```python
from build123d import *

# Parameters (mm, degrees)
F0_W      = 68.1
F0_H      = 138.3
F1_DEPTH  = 5.08
F2_R      = 8.93259
F3_T      = -1.15
F4_W      = 24.09836
F4_H      = 13.196725
F5_DEPTH  = 12.5
F6_W      = 48.097777
F6_H      = 7.753484
F7_DEPTH  = 12.5
F8_W      = 10.118616
F8_H      = 41.666549
F9_DEPTH  = 12.5
F10_W     = 6.856616
F10_H     = 19.977162
F11_DEPTH = 12.5
F12_SIZE  = 5


with BuildPart() as f1:
    # F0 (on Front) → F1 (new body, symmetric)
    with BuildSketch(Plane.XZ):
        Rectangle(F0_W, F0_H)
    extrude(amount=F1_DEPTH, both=True)

    # F2
    f2_edges = [f1.edges().sort_by_distance(p)[0] for p in [
        (-34.05, 0, 69.15),
        (34.05, 0, 69.15),
        (34.05, 0, -69.15),
        (-34.05, 0, -69.15),
    ]]
    fillet(f2_edges, radius=F2_R)

    # F3
    f3_openings = [f1.faces().sort_by_distance(p)[0] for p in [
        (0, -5.08, 0),
    ]]
    offset(amount=F3_T, openings=f3_openings)

    # F4 (on face) → F5 (cut, symmetric)
    with BuildSketch(Plane.XZ):
        with Locations((15.348363, 59.815576)):
            Rectangle(F4_W, F4_H)
    extrude(amount=F5_DEPTH, both=True, mode=Mode.SUBTRACT)

    # F6 (on face) → F7 (cut, symmetric)
    with BuildSketch(Plane(origin=(0, 0, -69.15), x_dir=(1, 0, 0), z_dir=(0, 0, -1))):
        with Locations((0.003194, 0.064824)):
            Rectangle(F6_W, F6_H)
    extrude(amount=F7_DEPTH, both=True, mode=Mode.SUBTRACT)

    # F8 (on face) → F9 (cut, symmetric)
    with BuildSketch(Plane(origin=(-34.05, 0, 0), x_dir=(0, -1, 0), z_dir=(-1, 0, 0))):
        with Locations((3.675346, 37.227889)):
            Rectangle(F8_W, F8_H)
    extrude(amount=F9_DEPTH, both=True, mode=Mode.SUBTRACT)

    # F10 (on face) → F11 (cut, symmetric)
    with BuildSketch(Plane.YZ.offset(34.05)):
        with Locations((-1.651692, 39.359077)):
            Rectangle(F10_W, F10_H)
    extrude(amount=F11_DEPTH, both=True, mode=Mode.SUBTRACT)

    # F12
    f12_edges = [f1.edges().sort_by_distance(p)[0] for p in [
        (3.299183, 4.505, 66.413939),
        (27.397543, 4.505, 66.413939),
        (27.397543, 4.505, 53.217214),
        (3.299183, 4.505, 53.217214),
    ]]
    chamfer(f12_edges, length=F12_SIZE)


solid = f1.part
```
Geometry check sheet. Reference: the model listing, model coordinates, mm. A direction names the side the tool comes from. Give positions to 0.01 mm unless a question says otherwise; leave off trailing zeros. Write each loop counter-clockwise with the first axis right and the second up, starting at its lowest first coordinate (ties: lowest second). Pieces come first, ordered by that corner, then holes. Notation, with made-up numbers: (2.25, 11.25) - (48.25, 11.25) arc R17 ccw to (48.25, 42.25) - close; hole circle Ø5 at (43.25, 46). An arc over 180 degrees is marked (long way). Use a Markdown table: item, result.
Q1. Thickness scan on L1, parallel to X at y = 2.25, z = 2; L2, parallel to Z at x = 15, y = -1.75; L3, parallel to Y at x = 10.5, z = 48. Record the ranges inside material, lowest first. Write a range as [from, to].
Computed:
| item | result |
|---|---|
| L1 | x = [-34.05, -32.9], [32.9, 34.05] |
| L2 | z = [68, 69.15] |
| L3 | y = [3.93, 5.08] |
Q2. Section check B-B, the plane x = -19. Enter the section's corners in (y, z), then the cut area to 3 significant figures.
Computed:
| item | result |
|---|---|
| outline | (-5.08, -69.15) - (-3.94, -69.15) - (-3.94, -68) - (-5.08, -68) - close; (-5.08, 68) - (3.93, 68) - (3.93, -68) - (3.81, -68) - (3.81, -69.15) - (5.08, -69.15) - (5.08, 69.15) - (-5.08, 69.15) - close |
| area | 171 mm² |
Q3. Section check D-D, the plane z = -39.5. Enter the section's corners in (x, y), then the cut area to 3 significant figures.
Computed:
| item | result |
|---|---|
| outline | (-34.05, -5.08) - (-32.9, -5.08) - (-32.9, 3.93) - (32.9, 3.93) - (32.9, -5.08) - (34.05, -5.08) - (34.05, 5.08) - (-34.05, 5.08) - close |
| area | 99.0 mm² |
Q4. Go/stop test with flat-tipped pins: P1, Ø0.9, axis at x = -33.5, y = -0.5, coming from the -Z side; P2, Ø0.9, axis at x = -33.5, z = 47.5, coming from the -Y side; P3, Ø1.3, axis at y = 4.5, z = 60.5, coming from the +X side; P4, Ø0.6, axis at x = 33.5, z = 40, coming from the -Y side. Record where each tip stops, or that it passes through.
Computed:
| item | result |
|---|---|
| P1 | stops at z = -64.32 |
| P2 | stops at y = 1.38 |
| P3 | stops at x = 34.05 |
| P4 | stops at y = 1.78 |
Q5. Draft check along X on faces 4 (the face through (0, 3.93, 1)), 5 (the face through (24.93, 4.51, 55.75)), 6 (the face through (-0.1, -4.2, -69.15)), 7 (the face through (-31.503, -0.071, -66.464)). Enter one of: pulls with the +X half, pulls with the -X half, needs draft (parallel to the pull), parting line crosses it, or undercut.
Computed:
| item | result |
|---|---|
| face 4 | undercut |
| face 5 | undercut |
| face 6 | needs draft |
| face 7 | pulls with the -X half |
Q6. Section check A-A, the plane y = -1.5. Enter the section's corners in (x, z), then the cut area to 3 significant figures.
Computed:
| item | result |
|---|---|
| outline | (-34.05, -60.22) arc R8.93 ccw to (-25.12, -69.15) - (-24.05, -69.15) - (-24.05, -68) - (-25.12, -68) arc R7.78 cw to (-32.9, -60.22) - (-32.9, 16.39) - (-34.05, 16.39) - close; (-34.05, 58.06) - (-32.9, 58.06) - (-32.9, 60.22) arc R7.78 cw to (-25.12, 68) - (25.12, 68) arc R7.78 cw to (32.9, 60.22) - (32.9, 49.35) - (34.05, 49.35) - (34.05, 60.22) arc R8.93 ccw to (25.12, 69.15) - (-25.12, 69.15) arc R8.93 ccw to (-34.05, 60.22) - close; (24.05, -69.15) - (25.12, -69.15) arc R8.93 ccw to (34.05, -60.22) - (34.05, 29.37) - (32.9, 29.37) - (32.9, -60.22) arc R7.78 cw to (25.12, -68) - (24.05, -68) - close |
| area | 327 mm² |
Q7. Set-up check for faces 1 (the face through (24.86, 4.5, 63.95)), 2 (the face through (0, 5.08, 1)), 3 (the face through (30.68, -0.51, 65.66)): record each of +Z, -Z, +X, -X, +Y, -Y from which the full face is reachable in a straight line by a thin tool's end or side.
Computed:
| item | result |
|---|---|
| face 1 | +Y, -Y |
| face 2 | +Z, -Z, +X, -X, +Y |
| face 3 | -Y |
Q8. Section check C-C, the plane x = 11. Enter the section's corners in (y, z).
Computed:
| item | result |
|---|---|
| outline | (-5.08, -69.15) - (-3.94, -69.15) - (-3.94, -68) - (-5.08, -68) - close; (-5.08, 68) - (3.93, 68) - (3.93, 66.41) - (5.08, 66.41) - (5.08, 69.15) - (-5.08, 69.15) - close; (3.81, -69.15) - (5.08, -69.15) - (5.08, 53.22) - (3.93, 53.22) - (3.93, -68) - (3.81, -68) - close |
